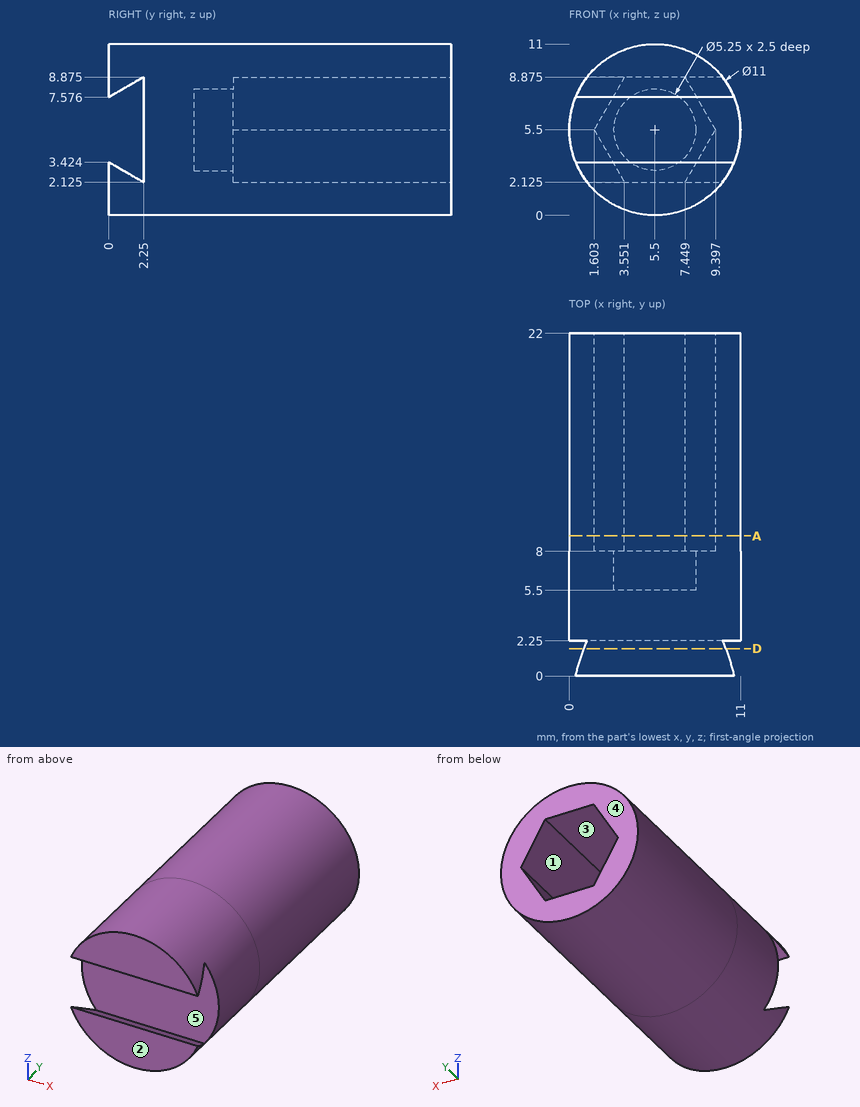
Check sheet for the drawn part. Datum: minimum x, y, z corner. Units: mm. A direction names the side the tool comes from. Round coordinates to 2 decimals unless told otherwise and drop trailing zeros. Write each loop counter-clockwise with the first axis right and the second up, starting at its lowest first coordinate (ties: lowest second). Pieces come first, ordered by that corner, then holes. Notation, with made-up numbers: (83, -33) - (102, -33) arc R21 ccw to (102, 5) - close; hole circle Ø1 at (13.25, 49.25). An arc over 180 degrees is marked (long way). Write each question's results on one line, items separated by ' | '.
(1) Set-up check for the marked faces 3, 4 and 5: record each of +Z, -Z, +X, -X, +Y, -Y from which the full face is reachable in a straight line by a thin tool's end or side.
Computed:
face 3: +Y | face 4: +Z, -Z, +X, -X, +Y | face 5: +X, -X
(2) Draft check along Z on the marked faces 1 and 2. Enter one of: pulls with the +Z half, pulls with the -Z half, needs draft (parallel to the pull), parting line crosses it, or undercut.
Computed:
face 1: undercut | face 2: needs draft
(3) Sectioned sample at D-D, the plane y = 1.75. Enter the section's corners in (x, z), plus the area to 3 significant figures.
Computed:
outline: (0.95, 2.41) arc R5.5 ccw to (10.05, 2.41) - close; (0.95, 8.59) - (10.05, 8.59) arc R5.5 ccw to start | area: 30.9 mm^2
(4) Sectioned sample at A-A, the plane y = 9. Enter the section's corners in (x, z) (1 decimal).
Computed:
outline: circle Ø11 at (5.5, 5.5); hole (1.6, 5.5) - (3.6, 2.1) - (7.4, 2.1) - (9.4, 5.5) - (7.4, 8.9) - (3.6, 8.9) - close
(5) Thickness scan on probe 1 along X at (y, z) = (7, 5.5) (1 decimal); probe 2 along Y at (x, z) = (1.5, 2.5); probe 3 along Y at (x, z) = (6.75, 7.5). Record the ranges inside material, lowest first. Write a range as from..to.
Computed:
probe 1: x = 0..2.9, 8.1..11 | probe 2: y = 0..1.6, 2.25..22 | probe 3: y = 2.25..5.5
(6) Depth check by flat-ended pin: pin 1 Ø3 at (y, z) = (19.5, 7.5) entering from -X; pin 2 Ø2 at (x, z) = (4, 5) entering from -Y; pin 3 Ø1.5 at (y, z) = (11, 2) entering from -X. Enter the tip coordinate at first touch or a pass-through.
Computed:
pin 1: stops at x = 0.02 | pin 2: stops at y = 2.25 | pin 3: stops at x = 0.74
